```python
from build123d import *

# Parameters (mm, degrees)
SKETCH1_R           = 1.2
BOSS_EXTRUDE1_DEPTH = 1.9
SKETCH2_W           = 1.3
SKETCH2_H           = 4.38685961
SKETCH2_R           = 0.96
BOSS_EXTRUDE2_DEPTH = 8
SKETCH3_W           = 9.6
SKETCH3_H           = 8.897442439
BOSS_EXTRUDE3_DEPTH = 6.7


with BuildPart() as part:
    # Sketch1 → Boss-Extrude1 (new body)
    with BuildSketch(Plane(origin=(0, 0, 0), x_dir=(1, 0, 0), z_dir=(0, 1, 0))):
        with BuildLine():
            Line((-5.55, 4.45), (5.55, 4.45))
            ThreePointArc((5.55, 4.45), (8.661269837, 3.161269837), (9.95, 0.05))
            Line((9.95, 0.05), (9.95, -0.05))
            ThreePointArc((9.95, -0.05), (8.661269837, -3.161269837), (5.55, -4.45))
            Line((5.55, -4.45), (-5.55, -4.45))
            ThreePointArc((-5.55, -4.45), (-8.661269837, -3.161269837), (-9.95, -0.05))
            Line((-9.95, -0.05), (-9.95, 0.05))
            ThreePointArc((-9.95, 0.05), (-8.661269837, 3.161269837), (-5.55, 4.45))
        make_face()
        with Locations((-7.7, 0)):
            Circle(SKETCH1_R, mode=Mode.SUBTRACT)
        with Locations((7.7, 0)):
            Circle(SKETCH1_R, mode=Mode.SUBTRACT)
    extrude(amount=BOSS_EXTRUDE1_DEPTH)

    # Sketch2 → Boss-Extrude2 (add)
    with BuildSketch(Plane(origin=(0, 1.9, 0), x_dir=(1, 0, 0), z_dir=(0, 1, 0))):
        with BuildLine():
            Line((1.3, 4.45), (-5.55, 4.45))
            ThreePointArc((-5.55, 4.45), (-5.625010901, 4.449360563), (-5.7, 4.447442439))
            Line((-5.7, 4.447442439), (-5.7, -4.447442439))
            ThreePointArc((-5.7, -4.447442439), (-5.625010901, -4.449360563), (-5.55, -4.45))
            Line((-5.55, -4.45), (1.3, -4.45))
            ThreePointArc((1.3, -4.45), (4.411269837, -3.161269837), (5.7, -0.05))
            Line((5.7, -0.05), (5.7, 0.05))
            ThreePointArc((5.7, 0.05), (4.411269837, 3.161269837), (1.3, 4.45))
        make_face()
        with BuildLine():
            Line((-4.55, -3.3), (-4.55, 3.3))
            Line((-4.55, 3.3), (1.3, 3.3))
            ThreePointArc((1.3, 3.3), (3.598097039, 2.348097039), (4.55, 0.05))
            Line((4.55, 0.05), (4.55, -0.05))
            ThreePointArc((4.55, -0.05), (3.598097039, -2.348097039), (1.3, -3.3))
            Line((1.3, -3.3), (-4.55, -3.3))
        make_face(mode=Mode.SUBTRACT)
        with Locations((-2.99802734, 0)):
            Rectangle(SKETCH2_W, SKETCH2_H)
        with Locations((1.3, 0)):
            Circle(SKETCH2_R)
    extrude(amount=BOSS_EXTRUDE2_DEPTH)

    # Sketch3 → Boss-Extrude3 (add)
    with BuildSketch(Plane.XZ):
        with Locations((-0.9, 0.00127878)):
            Rectangle(SKETCH3_W, SKETCH3_H)
    extrude(amount=BOSS_EXTRUDE3_DEPTH)


solid = part.part
```
Here's how the part is built. I have some questions about the finished solid (model axes, mm). A direction names the side the tool comes from. Round coordinates to 2 decimals unless told otherwise and drop trailing zeros. Order: outer loops, then holes, each group sorted by start corner. A loop starts at its lowest first (then second) coordinate and runs counter-clockwise, first axis right, second up. Notation, with made-up numbers: M 45.25,35.25 L 84.25,35.25 A13 cw 84.25,55.25 Z; hole C -23,86 d6. An arc over 180 degrees is marked long. Use CSV: the item, a comma, the result in double quotes.
1) I want a section at A-A (y = 4.25). List the corners of the cut face in (x, z) for me, then the cut area to 3 significant figures.
Taken from the geometry:
outline,"M -5.7,-4.45 A4.4 ccw -5.55,-4.45 L 1.3,-4.45 A4.4 ccw 5.7,-0.05 L 5.7,0.05 A4.4 ccw 1.3,4.45 L -5.55,4.45 A4.4 ccw -5.7,4.45 Z; M -3.65,-2.19 L -2.35,-2.19 L -2.35,2.19 L -3.65,2.19 Z; C 1.3,0 d1.92; hole M -4.55,-3.3 L 1.3,-3.3 A3.25 ccw 4.55,-0.05 L 4.55,0.05 A3.25 ccw 1.3,3.3 L -4.55,3.3 Z"
area,"46.2 mm^2"
2) I want a section at C-C (y = 1.25). List the corners of the cut face in (x, z) for me, then the cut area to 3 significant figures.
Taken from the geometry:
outline,"M -9.95,-0.05 A4.4 ccw -5.55,-4.45 L 5.55,-4.45 A4.4 ccw 9.95,-0.05 L 9.95,0.05 A4.4 ccw 5.55,4.45 L -5.55,4.45 A4.4 ccw -9.95,0.05 Z; hole C -7.7,0 d2.4; hole C 7.7,0 d2.4"
area,"151 mm^2"
3) If we mould it in two halves opening along Z, with no side actions, what happens to faces 1 (the flat face through (-1, -3, -4.447)), 2 (the flat face through (-5.7, 6, 0)), 3 (the cylindrical face through (3.573, 5.844, -2.373))? For each: pulls with the +Z half, pulls with the -Z half, needs draft (parallel to the pull), parting line crosses it, or undercut.
Taken from the geometry:
face 1,"pulls with the -Z half"
face 2,"needs draft"
face 3,"undercut"
4) I want a section at D-D (x = -7.5). List the corners of the cut face in (y, z) for me, then the cut area to 3 significant figures.
Taken from the geometry:
outline,"M 0,-3.99 L 1.9,-3.99 L 1.9,-1.18 L 0,-1.18 Z; M 0,1.18 L 1.9,1.18 L 1.9,3.99 L 0,3.99 Z"
area,"10.7 mm^2"
5) I need wall thicknesses on line 1 along X through (y, z) = (1.1, 0); line 2 along X through (y, z) = (2.75, -1.5); line 3 along X through (y, z) = (6, -0.75). Which ranges of each line are inside material? Lowest first, please. Write a range as [from, to].
Taken from the geometry:
line 1,"[-9.95, -8.9], [-6.5, 6.5], [8.9, 9.95]"
line 2,"[-5.7, -4.55], [-3.65, -2.35], [4.21, 5.45]"
line 3,"[-5.7, -4.55], [-3.65, -2.35], [0.7, 1.9], [4.47, 5.64]"
6) I'm going to push flat-ended pins straight in: P1, Ø2, axis at x = -6.5, y = 2.5, coming from the -Z side; P2, Ø1.9, axis at x = -7.7, z = 0, coming from the +Y side; P3, Ø2.5, axis at y = 4.5, z = -0.5, coming from the -X side; P4, Ø5.5, axis at x = -2, y = -3, coming from the -Z side. Where does each tip first touch, or does it pass through?
Taken from the geometry:
P1,"z = -4.45"
P2,"through"
P3,"x = -5.7"
P4,"z = -4.45"
7) On a 3-axis mill with a long thin cutter (end or side, diameter ignored), from which of +Z, -Z, +X, -X, +Y, -Y can I reach the whole of each face in a straight line? I mean faces 4 (the cylindrical face through (2.216, 5.844, -0.288)), 5 (the flat face through (6.6, 1.9, 0.9)), 6 (the flat face through (-5.7, -3, 0)). Say none if no direction works.
Taken from the geometry:
face 4,"+Y"
face 5,"+X, +Y"
face 6,"+Z, -Z, -X, -Y"
